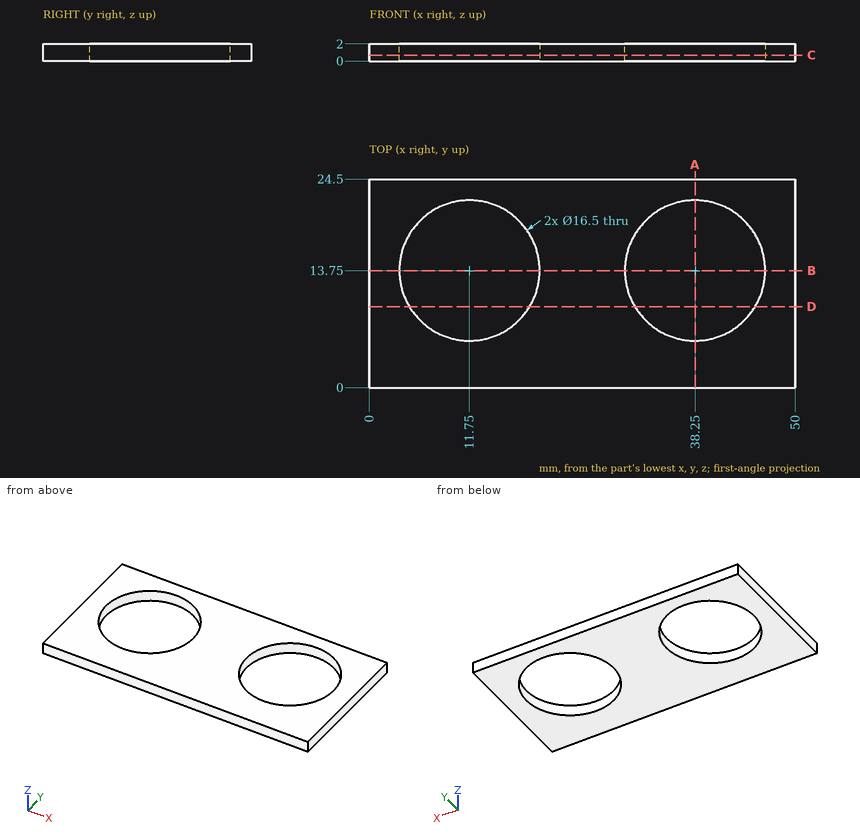
Geometry: see drawing. Coordinates: mm, zero at the bounding-box minimum. Give positions to 0.01 mm unless a question says otherwise; leave off trailing zeros. Order: outer loops, then holes, each group sorted by start corner. A loop starts at its lowest first (then second) coordinate and runs counter-clockwise, first axis right, second up. Notation, with made-up numbers: (-4.5, 83.25) -> (43.5, 83.25) arc R12 cw to (43.5, 92.25) -> close; hole circle Ø11 at (-12, 67). An arc over 180 degrees is marked (long way). Write item = value, one per line.
Q1. Cut plane C-C, the plane z = 0.7. Output: boundary loops of the cut face in (x, y).
Data:
outline = (0, 0) -> (50, 0) -> (50, 24.5) -> (0, 24.5) -> close; hole circle Ø16.5 at (11.75, 13.75); hole circle Ø16.5 at (38.25, 13.75)
Q2. Cut plane B-B, the plane y = 13.75. Output: boundary loops of the cut face in (x, z), and give its area (3 significant figures).
Data:
outline = (0, 0) -> (3.5, 0) -> (3.5, 2) -> (0, 2) -> close; (20, 0) -> (30, 0) -> (30, 2) -> (20, 2) -> close; (46.5, 0) -> (50, 0) -> (50, 2) -> (46.5, 2) -> close
area = 34.0 mm^2
Q3. Cut plane D-D, the plane y = 9.5. Output: boundary loops of the cut face in (x, z), and give its area (3 significant figures).
Data:
outline = (0, 0) -> (4.68, 0) -> (4.68, 2) -> (0, 2) -> close; (18.82, 0) -> (31.18, 0) -> (31.18, 2) -> (18.82, 2) -> close; (45.32, 0) -> (50, 0) -> (50, 2) -> (45.32, 2) -> close
area = 43.4 mm^2
Q4. Material intervals for line 1 (X direction, y = 13.5, z = 1.8); line 2 (Y direction, x = 38.25, z = 0.8); line 3 (X direction, y = 17, z = 1.85), sorted ascending. Write a range as from..to.
Data:
line_1 = 0..3.5, 20..30, 46.5..50
line_2 = 0..5.5, 22..24.5
line_3 = 0..4.17, 19.33..30.67, 45.83..50
Q5. Cut plane A-A, the plane x = 38.25. Output: boundary loops of the cut face in (y, z).
Data:
outline = (0, 0) -> (5.5, 0) -> (5.5, 2) -> (0, 2) -> close; (22, 0) -> (24.5, 0) -> (24.5, 2) -> (22, 2) -> close
